```python
from build123d import *

# Parameters (mm, degrees)
ESTRUSIONE_ESTRUSIONE1_DEPTH = 18
SMUSSO1_SIZE                 = 0.7


with BuildPart() as part:
    # Schizzo1 → Estrusione-Estrusione1 (new body)
    with BuildSketch(Plane.XY):
        with BuildLine():
            Line((0, 16), (98, 16))
            ThreePointArc((98, 16), (114, 0), (98, -16))
            Line((98, -16), (0, -16))
            ThreePointArc((0, -16), (-16, 0), (0, 16))
        make_face()
    extrude(amount=ESTRUSIONE_ESTRUSIONE1_DEPTH)

    # Smusso1
    smusso1_edges = [part.edges().sort_by_distance(p)[0] for p in [
        (114, 0, 18),
        (49, 16, 18),
        (-16, 0, 18),
        (49, 16, 0),
        (114, 0, 0),
        (49, -16, 0),
        (-16, 0, 0),
        (49, -16, 18),
    ]]
    chamfer(smusso1_edges, length=SMUSSO1_SIZE)


solid = part.part
```
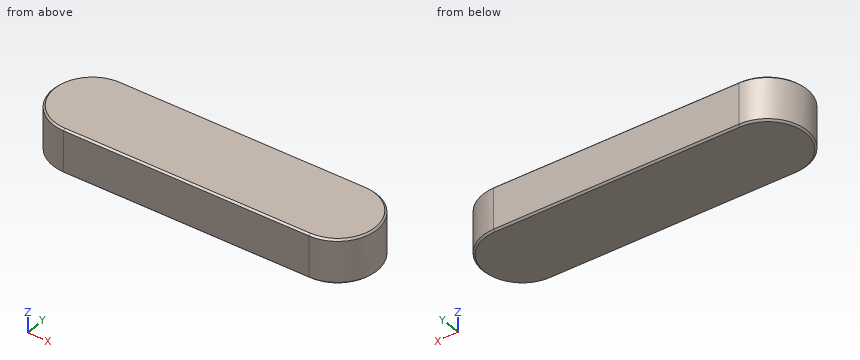
The model under review builds one solid part; all positions refer to its coordinate system, in mm. Coordinates: 2 decimals unless noted, no trailing zeros. Order: outer loops, then holes, each group sorted by start corner. A loop starts at its lowest first (then second) coordinate and runs counter-clockwise, first axis right, second up. Notation, with made-up numbers: M 20,-27 L 67,-27 A29 cw 67,8 Z; hole C 34.25,5.5 d10. An arc over 180 degrees is marked long. One line per question, with ' | ' between items.
(1) Insertion check: pin 1 (1 mm diameter, centred on y = -12.5, z = 12, fed in from +X); pin 2 (1 mm diameter, centred on y = -6, z = 8, fed in from +X) (3 decimals); pin 3 (10 mm diameter, centred on y = 7, z = 9, fed in from -X). Each pin has a flat end and moves straight along its axis. Give the tip position at first contact, or say it passes through.
Geometry results:
pin 1: stops at x = 108.58 | pin 2: stops at x = 113.025 | pin 3: stops at x = -15.87
(2) For probe 1 along X at (y, z) = (1.5, 11.25); probe 2 along Y at (x, z) = (-1.5, 8.5); probe 3 along Y at (x, z) = (-5, 6.5), list the stretches that pass through material, from the lowest coordinate up. Write a range as from..to.
Geometry results:
probe 1: x = -15.93..113.93 | probe 2: y = -15.93..15.93 | probe 3: y = -15.2..15.2
(3) Add section A-A, the plane z = 10.75. Write out the cut boundary in (x, y).
Geometry results:
outline: M 0,-16 L 98,-16 A16 ccw 98,16 L 0,16 A16 ccw Z
